Autodesk Inventor part; units mm, degrees
ref_plane "YZ Plane" through (0, 0, 0) normal (1, 0, 0) x (0, 1, 0)
ref_plane "XZ Plane" through (0, 0, 0) normal (0, 1, 0) x (-1, 0, 0)
ref_plane "XY Plane" through (0, 0, 0) normal (0, 0, 1) x (1, 0, 0)
sketch "Sketch1" plane through (0, 0, 0) normal (0, 0, 1) x (1, 0, 0)
  circle A0 centre (0, 0) radius 8
  circle A1 centre (0, 6) radius 1.5
  dimension "d0" = 16
  dimension "d1" = 3
  dimension "d2" = 6
  dimension "d3" = 0
extrude "Extrusion1" add sketch "Sketch1" along normal blind 15 contours A0 | A1
extrude "Extrusion2" add sketch "Sketch1" against normal blind 3 contours A1
chamfer "Chamfer1" distance 1 angle 70 1 edges at (-1.5, 6, -3) measured on face at (-0.1505, 5.5836, -3)
pattern_circular "Circular Pattern1" count 4 over 360 about axis through (0, 0, 0) along (0, 0, 1) of "Extrusion2", "Chamfer1"
sketch "Sketch3" plane through (0, 0, 15) normal (0, 0, 1) x (1, 0, 0)
  circle A0 centre (0, 0) radius 10
  dimension "d17" = 20
extrude "Extrusion4" add sketch "Sketch3" along normal blind 10
sketch "Sketch2" plane through (0, 0, 0) normal (0, 0, -1) x (-1, 0, 0)
  circle A0 centre (0, 0) radius 1.25
  dimension "d14" = 2.5
extrude "Extrusion3" cut sketch "Sketch2" against normal through all
sketch "Sketch4" plane through (0, 0, 25) normal (0, 0, 1) x (1, 0, 0)
  circle A0 centre (0, 0) radius 2
  dimension "d20" = 4
extrude "Extrusion5" cut sketch "Sketch4" against normal blind 23
properties part number "Motor1Gear"
The listing builds one solid part. Answer for the finished solid, in the listing's coordinates (mm). A direction names the side the tool comes from. Coordinates: 2 decimals unless noted, no trailing zeros. Write each loop counter-clockwise with the first axis right and the second up, starting at its lowest first coordinate (ties: lowest second). Pieces come first, ordered by that corner, then holes. Notation, with made-up numbers: M -16,21.5 L 14,21.5 A5 ccw 14,30.5 Z; hole C -5.75,49 d10. An arc over 180 degrees is marked long. Put each result on its own line as item: value. Start each with the question number.
1. A cutting plane is placed at D-D on x = 6. Write down the section's boundary in (y, z), then the cut area to 3 significant figures.
2. Flat-ended cylindrical pins translate along their axes: P1, Ø10, axis at x = -7.5, z = 0, coming from the +Y side; P2, Ø4.5, axis at x = 0, y = 1, coming from the +Z side; P3, Ø3, axis at x = 0, y = 0, coming from the -Z side; P4, Ø1.5, axis at x = 0.5, z = 14, coming from the +Y side. Find the tip coordinate at first contact, or state that the pin passes through.
3. For a pull along X with two mould halves and no side action, classify faces 1 (the conical face through (0.194, -5.125, -1.912)), 2 (the flat face through (0, -6, -3)), 3 (the cylindrical face through (0, -2, 14)) as pulls with the +X half, pulls with the -X half, needs draft (parallel to the pull), parting line crosses it, or undercut.
4. A cutting plane is placed at A-A on y = 0. Write down the section's boundary in (x, z).
5. Consider line 1 (Y direction, x = 0, z = 1.3); line 2 (Z direction, x = 5.25, y = 4); line 3 (Z direction, x = -1.25, y = -8). Determine where each line is inside the solid, lowest interval first. Write a range as from..to.
6. Which of the six approach directions +Z, -Z, +X, -X, +Y, -Y give full straight-line access (tool end or side, diameter ignored) to faces 4 (the flat face through (1, 1, 2)), 5 (the flat face through (-0.1, 2.4, 25)), 6 (the cylindrical face through (-1.73, 7.81, 7.4))?
7. A cutting plane is placed at C-C on z = 6. Write down the section's boundary in (x, y).
Resolved:
1. outline: M -8,15 L -5.29,15 L -5.29,0 L -1.5,0 L -1.5,-0.25 L -0.5,-3 L 0.5,-3 L 1.5,-0.25 L 1.5,0 L 5.29,0 L 5.29,15 L 8,15 L 8,25 L -8,25 Z
1. area: 325 mm2
2. P1: stops at y = 7.6
2. P2: stops at z = 25
2. P3: stops at z = 0
2. P4: stops at y = 8
3. face 1: parting line crosses it
3. face 2: needs draft
3. face 3: undercut
4. outline: M -10,15 L -8,15 L -8,0 L -7.5,0 L -7.5,-0.25 L -6.5,-3 L -5.5,-3 L -4.5,-0.25 L -4.5,0 L -1.25,0 L -1.25,2 L -2,2 L -2,25 L -10,25 Z; M 1.25,0 L 4.5,0 L 4.5,-0.25 L 5.5,-3 L 6.5,-3 L 7.5,-0.25 L 7.5,0 L 8,0 L 8,15 L 10,15 L 10,25 L 2,25 L 2,2 L 1.25,2 Z
5. line 1: y = -8..-1.25, 1.25..8
5. line 2: z = 0..25
5. line 3: z = 15..25
6. face 4: +Z
6. face 5: +Z, +X, -X, +Y, -Y
6. face 6: -Z
7. outline: C 0,0 d16; hole C 0,0 d4
